Design review of the part built by this model. Coordinates are the model's own, in mm. A direction names the side the tool comes from. Give positions to 0.01 mm unless a question says otherwise; leave off trailing zeros. Order: outer loops, then holes, each group sorted by start corner. A loop starts at its lowest first (then second) coordinate and runs counter-clockwise, first axis right, second up. Notation, with made-up numbers: (-38, 81.5) -> (17, 81.5) arc R26 ccw to (17, 103.5) -> close; hole circle Ø8 at (24, 34). An arc over 180 degrees is marked (long way). Answer in a Markdown table with one row per item. Add a question column.
```python
from build123d import *

# Parameters (mm, degrees)
SKETCH1_R                             = 75
BLOCO_DEPTH                           = 27
SKETCH2_R                             = 9
FURO_CENTRAL_18_PASSANTE_DEPTH        = 110.448618082
SKETCH2_3_R                           = 9
ENCAIXE_DO_EIXO_DEPTH                 = 10
REBAIXO_FUROS_DE_FIXA_O_M4_AT_2_COUNT = 2
REBAIXO_FUROS_DE_FIXA_O_M4_AT_2_PITCH = 65
REBAIXO_FUROS_DE_FIXA_O_M4_AT_3_COUNT = 2
REBAIXO_FUROS_DE_FIXA_O_M4_AT_3_PITCH = 112.583302492
REBAIXO_FUROS_DE_FIXA_O_M4_AT_4_COUNT = 2
REBAIXO_FUROS_DE_FIXA_O_M4_AT_4_PITCH = 130
REBAIXO_FUROS_DE_FIXA_O_M4_AT_5_COUNT = 2
REBAIXO_FUROS_DE_FIXA_O_M4_AT_5_PITCH = 112.583302492
REBAIXO_FUROS_DE_FIXA_O_M4_AT_6_COUNT = 2
REBAIXO_FUROS_DE_FIXA_O_M4_AT_6_PITCH = 65
RASGO_DIMENSIONADO_DEPTH              = 110.448618082
RASGOS_COUNT                          = 5
SKETCH7_R                             = 4


with BuildPart() as part:
    # Sketch1 → Bloco (new body)
    with BuildSketch(Plane(origin=(0, 0, 0), x_dir=(1, 0, 0), z_dir=(0, 1, 0))):
        with Locations(Location((0, 0, 0), (0, 0, 270))):
            Circle(SKETCH1_R)
    extrude(amount=-BLOCO_DEPTH)

    # Sketch2 → Furo Central - _18 Passante (cut, through all)
    with BuildSketch(Plane(origin=(0, 0, 0), x_dir=(-1, 0, 0), z_dir=(0, 1, 0))):
        with Locations(Location((0, 0, 0), (0, 0, 90))):
            Circle(SKETCH2_R)
    extrude(amount=-FURO_CENTRAL_18_PASSANTE_DEPTH, mode=Mode.SUBTRACT)

    # Sketch2_3 → Encaixe do Eixo (cut)
    with BuildSketch(Plane(origin=(0, 0, 0), x_dir=(-1, 0, 0), z_dir=(0, 1, 0))):
        Polygon((-8.660254038, 15), (-17.320508076, 0), (-8.660254038, -15), (8.660254038, -15), (17.320508076, 0), (8.660254038, 15), align=None)
        with Locations(Location((0, 0, 0), (0, 0, 90))):
            Circle(SKETCH2_3_R, mode=Mode.SUBTRACT)
    extrude(amount=-ENCAIXE_DO_EIXO_DEPTH, mode=Mode.SUBTRACT)

    # Sketch5 → Rebaixo - Furos de Fixa_o M4 (revolve, cut)
    with BuildSketch(Plane(origin=(32.5, -27, -56.291651246), x_dir=(0, 0, -1), z_dir=(1, 0, 0))):
        Polygon((0, 0), (0, 27), (2.25, 27), (2.25, 4), (4, 4), (4, 0.025), (4.025, 0), align=None)
    rebaixo_furos_de_fixa_o_m4 = revolve(axis=Axis((32.5, -33.35, -56.291651246), (0, 1, 0)), mode=Mode.SUBTRACT)

    # Rebaixo - Furos de Fixa_o M4 at 2: Rebaixo - Furos de Fixa_o M4 ×2
    with Locations(*[(-i * REBAIXO_FUROS_DE_FIXA_O_M4_AT_2_PITCH, 0, 0) for i in range(1, REBAIXO_FUROS_DE_FIXA_O_M4_AT_2_COUNT)]):
        add(rebaixo_furos_de_fixa_o_m4, mode=Mode.SUBTRACT)

    # Rebaixo - Furos de Fixa_o M4 at 3: Rebaixo - Furos de Fixa_o M4 ×2
    with Locations(*[Vector(-0.866025403784438, 0, 0.5000000000000011) * (i * REBAIXO_FUROS_DE_FIXA_O_M4_AT_3_PITCH) for i in range(1, REBAIXO_FUROS_DE_FIXA_O_M4_AT_3_COUNT)]):
        add(rebaixo_furos_de_fixa_o_m4, mode=Mode.SUBTRACT)

    # Rebaixo - Furos de Fixa_o M4 at 4: Rebaixo - Furos de Fixa_o M4 ×2
    with Locations(*[Vector(-0.4999999999999989, 0, 0.8660254037844394) * (i * REBAIXO_FUROS_DE_FIXA_O_M4_AT_4_PITCH) for i in range(1, REBAIXO_FUROS_DE_FIXA_O_M4_AT_4_COUNT)]):
        add(rebaixo_furos_de_fixa_o_m4, mode=Mode.SUBTRACT)

    # Rebaixo - Furos de Fixa_o M4 at 5: Rebaixo - Furos de Fixa_o M4 ×2
    with Locations(*[(0, 0, i * REBAIXO_FUROS_DE_FIXA_O_M4_AT_5_PITCH) for i in range(1, REBAIXO_FUROS_DE_FIXA_O_M4_AT_5_COUNT)]):
        add(rebaixo_furos_de_fixa_o_m4, mode=Mode.SUBTRACT)

    # Rebaixo - Furos de Fixa_o M4 at 6: Rebaixo - Furos de Fixa_o M4 ×2
    with Locations(*[Vector(0.5000000000000009, 0, 0.8660254037844382) * (i * REBAIXO_FUROS_DE_FIXA_O_M4_AT_6_PITCH) for i in range(1, REBAIXO_FUROS_DE_FIXA_O_M4_AT_6_COUNT)]):
        add(rebaixo_furos_de_fixa_o_m4, mode=Mode.SUBTRACT)

    # Sketch6 → Rasgo Dimensionado (cut, through all)
    with BuildSketch(Plane(origin=(0, -27, 0), x_dir=(-1, 0, 0), z_dir=(0, -1, 0))):
        with BuildLine():
            ThreePointArc((-4.942704321, 30.754767512), (0, 25), (4.942704321, 30.754767512))
            ThreePointArc((4.942704321, 30.754767512), (5.310250702, 32.70762802), (6.817704321, 34.002362777))
            ThreePointArc((6.817704321, 34.002362777), (9.330127019, 41.160254038), (1.875, 42.563377787))
            ThreePointArc((1.875, 42.563377787), (0, 41.905252036), (-1.875, 42.563377787))
            ThreePointArc((-1.875, 42.563377787), (-9.330127019, 41.160254038), (-6.817704321, 34.002362777))
            ThreePointArc((-6.817704321, 34.002362777), (-5.310250702, 32.70762802), (-4.942704321, 30.754767512))
        make_face()
    rasgo_dimensionado = extrude(amount=-RASGO_DIMENSIONADO_DEPTH, mode=Mode.SUBTRACT)

    # Rasgos: Rasgo Dimensionado ×5 about axis
    rasgos_axis = Axis((0, 0, 0), (0, 1, 0))
    for i in range(1, RASGOS_COUNT):
        add(rasgo_dimensionado.rotate(rasgos_axis, i * 360 / RASGOS_COUNT), mode=Mode.SUBTRACT)

    # Sketch7 → Canal - Raio de 4mm (revolve, cut)
    with BuildSketch(Plane(origin=(0, 0, 0), x_dir=(0, 0, -1), z_dir=(1, 0, 0)), mode=Mode.PRIVATE) as canal_raio_de_4mm_sk:
        with Locations((-53.5, -27)):
            Circle(SKETCH7_R)
    revolve(canal_raio_de_4mm_sk.sketch.rotate(Axis((0, -27, 0), (0, 1, 0)), 180), axis=Axis((0, -27, 0), (0, 1, 0)), mode=Mode.SUBTRACT)


solid = part.part
```
1) Add section C-C, the plane z = 62.5. Write out the cut boundary in (x, y).
2) Add section A-A, the plane x = -65. Write out the cut boundary in (y, z) (3 decimals), and give its area (4 significant figures).
3) Mouldability with a two-part tool opening along Z and no side actions: class faces 1 (the face through (-45.636, -13.311, -59.517)), 2 (the face through (-36.38, -13.689, -21.566)) as +Z half, -Z half, draft (parallel to the pull), parting line (faces both ways), or undercut.
4) Clearance check with flat-ended pins moving along their axes: P1, Ø13, axis at x = -35.22, z = -16.7, coming from the +Y side; P2, Ø7, axis at x = -65, z = 0, coming from the -Y side; P3, Ø4, axis at y = -13.5, z = 56, coming from the -X side; P4, Ø8, axis at x = -22, y = -8.5, coming from the +Z side. State where each tip first meets the part, or that it passes through.
5) Add section B-B, the plane y = -25. Give the number of separate pieces and of enclosed holes in the cut face, and give its area (3 significant figures).
6) For L1, parallel to X at y = -15.5, z = 0; L2, parallel to X at y = -8.5, z = -8.5; L3, parallel to Z at x = 39, y = -24.25, list the stretches that pass through material, from the lowest coordinate up.
7) Machinability: for faces 3 (the face through (14.93, -13.69, 29.61)), 4 (the face through (-30.78, -23, -54.57)), 5 (the face through (12.93, -4.93, 7.605)), which of the approach directions +Z, -Z, +X, -X, +Y, -Y give a long, thin tool a straight path to every point of the face, cutting with its end or side? Answer none if there is none.
Verdict:
| question | item | result |
|---|---|---|
| 1 | outline | (-41.46, -27) -> (41.46, -27) -> (41.46, 0) -> (-41.46, 0) -> close |
| 2 | outline | (-27, -37.417) -> (0, -37.417) -> (0, -2.25) -> (-23, -2.25) -> (-23, -4) -> (-26.975, -4) -> (-27, -4.025) -> close; (-27, 4.025) -> (-26.975, 4) -> (-23, 4) -> (-23, 2.25) -> (0, 2.25) -> (0, 37.417) -> (-27, 37.417) -> close |
| 2 | area | 1,885 mm2 |
| 3 | face 1 | parting line |
| 3 | face 2 | undercut |
| 4 | P1 | stops at y = 0 |
| 4 | P2 | stops at y = -23 |
| 4 | P3 | stops at x = -52.05 |
| 4 | P4 | stops at z = 72.81 |
| 5 | separate pieces | 2 |
| 5 | enclosed holes | 13 |
| 5 | area | 13,500 mm2 |
| 6 | L1 | x = -75 to -67.25, -62.75 to -9, 9 to 62.75, 67.25 to 75 |
| 6 | L2 | x = -74.52 to -43.14, -23.59 to -12.41, 12.41 to 23.59, 43.14 to 74.52 |
| 6 | L3 | z = -64.06 to -40.75, -32.23 to -19.98, -2.24 to 32.23, 40.75 to 64.06 |
| 7 | face 3 | +Y, -Y |
| 7 | face 4 | -Y |
| 7 | face 5 | +Y |
